The listing builds one solid part. Answer for the finished solid, in the listing's coordinates (mm). Face numbers are marked on the shaded views. A direction names the side the tool comes from. Coordinates: 2 decimals unless noted, no trailing zeros. Order: outer loops, then holes, each group sorted by start corner. A loop starts at its lowest first (then second) coordinate and runs counter-clockwise, first axis right, second up. Notation, with made-up numbers: (81.25, -5) - (89.25, -5) arc R18 cw to (89.25, 24) - close; hole circle Ø6 at (56.5, 9.25). An arc over 180 degrees is marked (long way). Use a Markdown table: item, result. Add a question column.
Item 1: The part is cut by section B-B, the plane x = -24. Give the vertices of the cut face in (y, z).
Item 2: For the marked faces 1, 2 and 3, determine the directions among +Z, -Z, +X, -X, +Y, -Y from which every point of the face is accessible in a straight line to the end or side of a thin tool.
Item 3: The part is cut by section A-A, the plane z = 34. Give the vertices of the cut face in (x, y), then the cut area to 3 significant figures.
Item 4: The part is cut by section D-D, the plane y = 10.5. Give the vertices of the cut face in (x, z), then the cut area to 3 significant figures.
Item 5: The mould has two halves that part along Y. Classify the marked faces 4, 5 and 6: released by +Y, released by -Y, zero draft, split by the parting line, or undercut.
Item 6: The part is cut by section C-C, the plane z = 7. Give the vertices of the cut face in (x, y).
Item 7: Flat-ended cylindrical pins translate along their axes: P1, Ø8, axis at x = -19, z = 10.5, coming from the -Y side; P2, Ø2, axis at x = 7.5, y = -5, coming from the -Z side; P3, Ø11, axis at x = -21.37, y = 0.45, coming from the -Z side; P4, Ø5.5, axis at y = 4.5, z = 31.5, coming from the -X side. Find the tip coordinate at first contact, or state that the pin passes through.
Item 8: Find the intervals of material crossed by line 1 along X through (y, z) = (2, 41.5); line 2 along Y through (x, z) = (-24, 3.5); line 3 along Y through (x, z) = (39, 4), in increasing order.
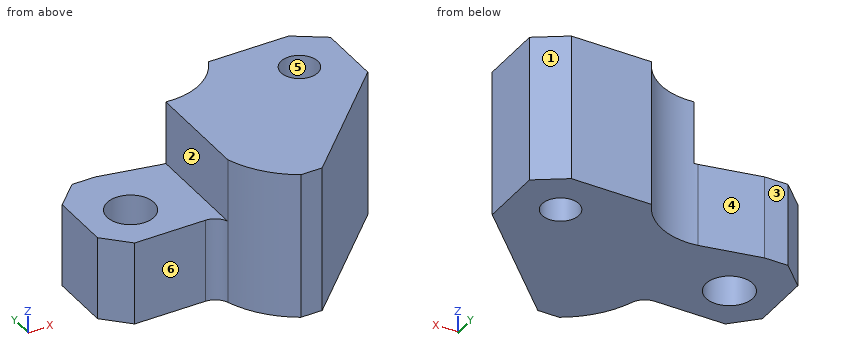
from build123d import *

# Parameters (mm, degrees)
F0_R     = 7
F0_R_2   = 5.5
F1_DEPTH = 44
F2_R     = 7
F3_DEPTH = 19


with BuildPart() as f1:
    # F0 (on Top) → F1 (new body)
    with BuildSketch(Plane.XY):
        with BuildLine():
            Line((-28.369482, 18.450219), (-35.369482, 11.450219))
            Line((-35.369482, 11.450219), (-35.369482, -6.549781))
            Line((-35.369482, -6.549781), (-28.369482, -13.549781))
            Line((-28.369482, -13.549781), (-7.182735, -13.549781))
            ThreePointArc((-7.182735, -13.549781), (-4.272748, -14.483828), (-2.449987, -16.936991))
            ThreePointArc((-2.449987, -16.936991), (2.500816, -25.88004), (10.246986, -32.549781))
            Line((10.246986, -32.549781), (16.630518, -32.549781))
            Line((16.630518, -32.549781), (49.630518, 0.450219))
            Line((49.630518, 0.450219), (49.630518, 19.450219))
            Line((49.630518, 19.450219), (40.630518, 25.450219))
            Line((40.630518, 25.450219), (16.630518, 25.450219))
            ThreePointArc((16.630518, 25.450219), (8.304904, 16.782132), (-3.55667, 14.844443))
            Line((-3.55667, 14.844443), (-21.369482, 18.450219))
            Line((-21.369482, 18.450219), (-28.369482, 18.450219))
        make_face()
        with Locations((-21.369482, 0.450219)):
            Circle(F0_R, mode=Mode.SUBTRACT)
        with Locations((35.630518, 11.450219)):
            Circle(F0_R_2, mode=Mode.SUBTRACT)
    extrude(amount=F1_DEPTH)

    # F2 (on face) → F3 (cut)
    with BuildSketch(Plane.XY.offset(44)):
        with BuildLine():
            Line((-2.449987, -16.936991), (-2.449987, 14.69919))
            ThreePointArc((-2.449987, 14.69919), (-3.004395, 14.763688), (-3.55667, 14.844443))
            Line((-3.55667, 14.844443), (-21.369482, 18.450219))
            Line((-21.369482, 18.450219), (-28.369482, 18.450219))
            Line((-28.369482, 18.450219), (-35.369482, 11.450219))
            Line((-35.369482, 11.450219), (-35.369482, -6.549781))
            Line((-35.369482, -6.549781), (-28.369482, -13.549781))
            Line((-28.369482, -13.549781), (-7.182735, -13.549781))
            ThreePointArc((-7.182735, -13.549781), (-4.272748, -14.483828), (-2.449987, -16.936991))
        make_face()
        with Locations((-21.369482, 0.450219)):
            Circle(F2_R, mode=Mode.SUBTRACT)
    extrude(amount=-F3_DEPTH, mode=Mode.SUBTRACT)


solid = f1.part
Solution:
| question | item | result |
|---|---|---|
| 1 | outline | (-13.55, 0) - (-6.04, 0) - (-6.04, 25) - (-13.55, 25) - close; (6.94, 0) - (18.45, 0) - (18.45, 25) - (6.94, 25) - close |
| 2 | face 1 | +Z, -Z, +X, +Y |
| 2 | face 2 | +Z, -X, +Y, -Y |
| 2 | face 3 | +Z, -Z, -X, +Y |
| 3 | outline | (-2.45, -16.94) arc R29 ccw to (10.25, -32.55) - (16.63, -32.55) - (49.63, 0.45) - (49.63, 19.45) - (40.63, 25.45) - (16.63, 25.45) arc R19 cw to (-2.45, 14.7) - close; hole circle Ø11 at (35.63, 11.45) |
| 3 | area | 2,130 mm2 |
| 4 | outline | (-35.37, 0) - (30.21, 0) - (30.21, 44) - (-2.45, 44) - (-2.45, 25) - (-35.37, 25) - close; (41.05, 0) - (49.63, 0) - (49.63, 44) - (41.05, 44) - close |
| 4 | area | 2,640 mm2 |
| 5 | face 4 | released by +Y |
| 5 | face 5 | undercut |
| 5 | face 6 | released by -Y |
| 6 | outline | (-35.37, -6.55) - (-28.37, -13.55) - (-7.18, -13.55) arc R5 cw to (-2.45, -16.94) arc R29 ccw to (10.25, -32.55) - (16.63, -32.55) - (49.63, 0.45) - (49.63, 19.45) - (40.63, 25.45) - (16.63, 25.45) arc R19 cw to (-3.56, 14.84) - (-21.37, 18.45) - (-28.37, 18.45) - (-35.37, 11.45) - close; hole circle Ø14 at (-21.37, 0.45); hole circle Ø11 at (35.63, 11.45) |
| 7 | P1 | stops at y = -13.55 |
| 7 | P2 | stops at z = 0 |
| 7 | P3 | passes through |
| 7 | P4 | stops at x = -2.45 |
| 8 | line 1 | x = -2.45 to 49.63 |
| 8 | line 2 | y = -13.55 to -6.04, 6.94 to 18.45 |
| 8 | line 3 | y = -10.18 to 7.1, 15.8 to 25.45 |
